Model file for the job. Use its own axes, mm. Face numbers are marked on the shaded views. Give positions to 0.01 mm unless a question says otherwise; leave off trailing zeros. Order: outer loops, then holes, each group sorted by start corner. A loop starts at its lowest first (then second) coordinate and runs counter-clockwise, first axis right, second up. Notation, with made-up numbers: (2, -23) - (49, -23) arc R15 ccw to (49, 5) - close; hole circle Ø9 at (21.25, 4). An arc over 180 degrees is marked (long way). Return JSON: item names as keys, results as strings. Group by question number.
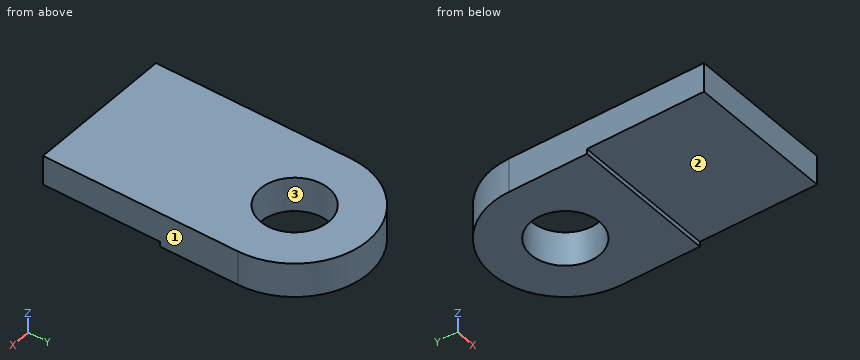
from build123d import *

# Parameters (mm, degrees)
SKETCH1_W           = 15
SKETCH1_H           = 12
BOSS_EXTRUDE1_DEPTH = 3
BOSS_EXTRUDE2_DEPTH = 3.5


with BuildPart() as part:
    # Sketch1 → Boss-Extrude1 (new body)
    with BuildSketch(Plane.XY):
        with Locations((7.5, 6)):
            Rectangle(SKETCH1_W, SKETCH1_H)
    extrude(amount=BOSS_EXTRUDE1_DEPTH)

    # Sketch2 → Boss-Extrude2 (add)
    with BuildSketch(Plane.XY.offset(3)):
        with BuildLine():
            Line((0, 20), (0, 12))
            Line((0, 12), (15, 12))
            Line((15, 12), (15, 20))
            ThreePointArc((15, 20), (7.5, 12.5), (0, 20))
        make_face()
        with BuildLine():
            ThreePointArc((15, 20), (7.5, 27.5), (0, 20))
            Line((0, 20), (4, 20))
            ThreePointArc((4, 20), (7.5, 23.5), (11, 20))
            Line((11, 20), (15, 20))
        make_face()
        with BuildLine():
            Line((4, 20), (0, 20))
            ThreePointArc((0, 20), (7.5, 12.5), (15, 20))
            Line((15, 20), (11, 20))
            ThreePointArc((11, 20), (7.5, 16.5), (4, 20))
        make_face()
    extrude(amount=-BOSS_EXTRUDE2_DEPTH)


solid = part.part
(1) Slice it at C-C (y = 9.25). Give the cut face in (x, z), and give its area (3 significant figures).
(2) Slice it at D-D (x = 9.25). Give the cut face in (y, z), and give its area (3 significant figures).
(3) Pull direction X, two halves, no side cores. Call the marked faces 1, 2 and 3: released by +X, released by -X, zero draft, split by the parting line, or undercut.
(4) Slice it at B-B (x = 1.5). Give the cut face in (y, z).
(5) Drill centre lines: L1, parallel to Y at x = 7.5, z = 0.9; L2, parallel to Z at x = 3.25, y = 8.5; L3, parallel to Y at x = 9.5, z = 1.3. Where is each one in solid material? Low to high.
(6) Slice it at A-A (x = 7.5). Give the cut face in (y, z).
Result set:
{
 "1": {"outline": "(0, 0) - (15, 0) - (15, 3) - (0, 3) - close", "area": "45.0 mm²"},
 "2": {"outline": "(0, 0) - (12, 0) - (12, -0.5) - (16.97, -0.5) - (16.97, 3) - (0, 3) - close; (23.03, -0.5) - (27.29, -0.5) - (27.29, 3) - (23.03, 3) - close", "area": "68.3 mm²"},
 "3": {"face 1": "released by +X", "face 2": "zero draft", "face 3": "undercut"},
 "4": {"outline": "(0, 0) - (12, 0) - (12, -0.5) - (24.5, -0.5) - (24.5, 3) - (0, 3) - close"},
 "5": {"L1": "y = 0 to 16.5, 23.5 to 27.5", "L2": "z = 0 to 3", "L3": "y = 0 to 17.13, 22.87 to 27.23"},
 "6": {"outline": "(0, 0) - (12, 0) - (12, -0.5) - (16.5, -0.5) - (16.5, 3) - (0, 3) - close; (23.5, -0.5) - (27.5, -0.5) - (27.5, 3) - (23.5, 3) - close"}
}
